Can you work these out from the drawing? Everything is in mm from the part's minimum corner. Round coordinates to 2 decimals unless told otherwise and drop trailing zeros. Order: outer loops, then holes, each group sorted by start corner. A loop starts at its lowest first (then second) coordinate and runs counter-clockwise, first axis right, second up. Notation, with made-up numbers: (7, 25.5) -> (20, 25.5) arc R15 ccw to (20, 41.5) -> close; hole circle Ø9 at (-14.5, 80). An arc over 180 degrees is marked (long way). One line per item, written item: value.
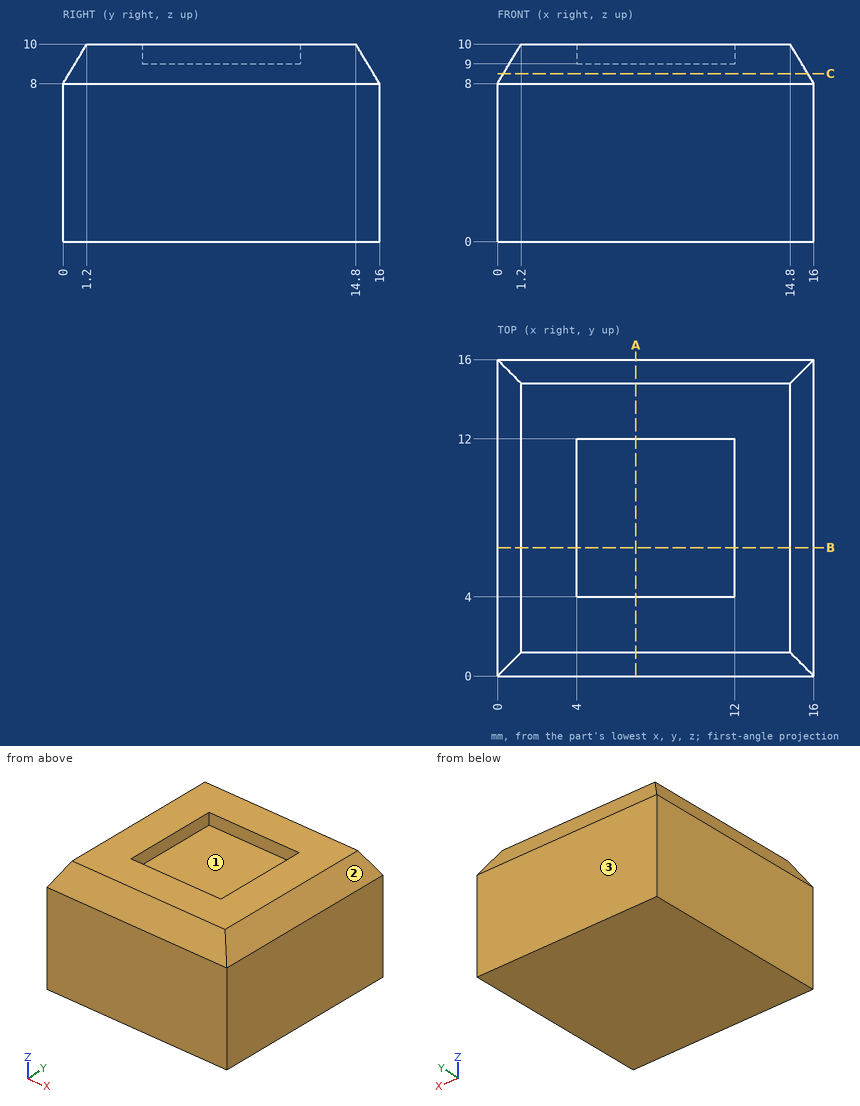
Q1. If we mould it in two halves opening along Y, with no side actions, what happens to the marked faces 1, 2 and 3? For each: pulls with the +Y half, pulls with the -Y half, needs draft (parallel to the pull), parting line crosses it, or undercut.
Answers:
face 1: undercut
face 2: needs draft
face 3: pulls with the +Y half
Q2. I want a section at A-A on x = 7. Write out the boundary of the cut face in (y, z), then the cut area to 3 significant figures.
Answers:
outline: (0, 0) -> (16, 0) -> (16, 8) -> (14.8, 10) -> (12, 10) -> (12, 9) -> (4, 9) -> (4, 10) -> (1.2, 10) -> (0, 8) -> close
area: 150 mm2
Q3. For P1, Ø1.5, axis at x = 13.5, y = 10, coming from the -Z side; P2, Ø0.5, axis at x = 9.5, z = 9.5, coming from the +Y side; P3, Ø0.8, axis at y = 8, z = 9.5, coming from the -X side; P4, Ø0.5, axis at x = 10, z = 9.5, coming from the -Y side, each with a flat end and sliding along its axis, tell me the tip position at first contact or that it passes through.
Answers:
P1: z = 0
P2: y = 15.25
P3: x = 0.66
P4: y = 0.75
Q4. I need wall thicknesses on line 1 along Z through (x, y) = (7.5, 5.5); line 2 along Y through (x, z) = (10, 9.75); line 3 along X through (y, z) = (4.5, 9.25). Which ranges of each line are inside material? Lowest first, please.
Answers:
line 1: 0 to 9
line 2: 1.05 to 4, 12 to 14.95
line 3: 0.75 to 4, 12 to 15.25
Q5. I want a section at C-C on z = 8.5. Write out the boundary of the cut face in (x, y).
Answers:
outline: (0.3, 0.3) -> (15.7, 0.3) -> (15.7, 15.7) -> (0.3, 15.7) -> close
